```python
from build123d import *

# Parameters (mm, degrees)
SKETCH1_W                      = 96
SKETCH1_H                      = 32
BOSS_EXTRUDE1_DEPTH            = 32
SKETCH2_W                      = 28
SKETCH2_H                      = 30
CUT_EXTRUDE1_DEPTH             = 97
F_8_0_8_DIAMETER_HOLE1_D       = 8
F_8_0_8_DIAMETER_HOLE1_DEPTH   = 2
F_3_7_3_7_DIAMETER_HOLE1_D     = 3.7
F_3_7_3_7_DIAMETER_HOLE1_DEPTH = 2
F_3_7_3_7_DIAMETER_HOLE2_D     = 3.7
F_3_7_3_7_DIAMETER_HOLE2_DEPTH = 32
F_8_0_8_DIAMETER_HOLE2_D       = 8
F_8_0_8_DIAMETER_HOLE2_DEPTH   = 32
F_8_0_8_DIAMETER_HOLE3_D       = 8
F_8_0_8_DIAMETER_HOLE3_DEPTH   = 2
F_8_0_8_DIAMETER_HOLE4_D       = 8
F_8_0_8_DIAMETER_HOLE4_DEPTH   = 32
F_3_7_3_7_DIAMETER_HOLE3_D     = 3.7
F_3_7_3_7_DIAMETER_HOLE3_DEPTH = 32
FILLET1_R                      = 2.5


with BuildPart() as part:
    # Sketch1 → Boss-Extrude1 (new body)
    with BuildSketch(Plane(origin=(16, 0, 0), x_dir=(0, 0, -1), z_dir=(1, 0, 0))):
        with Locations((32, 16)):
            Rectangle(SKETCH1_W, SKETCH1_H)
    extrude(amount=-BOSS_EXTRUDE1_DEPTH)

    # Sketch2 → Cut-Extrude1 (cut, through all)
    with BuildSketch(Plane(origin=(0, 0, -80), x_dir=(-1, 0, 0), z_dir=(0, 0, -1))):
        with Locations((0, 17)):
            Rectangle(SKETCH2_W, SKETCH2_H)
    extrude(amount=-CUT_EXTRUDE1_DEPTH, mode=Mode.SUBTRACT)

    # Ø8.0 (8) Diameter Hole1
    with Locations(Plane.ZY.offset(16)):
        with Locations((-64, 16), (-32, 16), (-16, 16), (-48, 16), (0, 16)):
            Hole(F_8_0_8_DIAMETER_HOLE1_D / 2, depth=F_8_0_8_DIAMETER_HOLE1_DEPTH)

    # Ø3.7 (3.7) Diameter Hole1
    with Locations(Plane.ZY.offset(16)):
        with Locations((0, 24), (0, 8), (-8, 16), (8, 16), (-5.656854249, 21.656854249), (5.656854249, 21.656854249), (5.656854249, 10.343145751), (-5.656854249, 10.343145751), (-64, 24), (-64, 8), (-72, 16), (-56, 16), (-69.656854249, 21.656854249), (-58.343145751, 21.656854249), (-58.343145751, 10.343145751), (-69.656854249, 10.343145751), (-32, 24), (-40, 16), (-32, 8), (-24, 16)):
            Hole(F_3_7_3_7_DIAMETER_HOLE1_D / 2, depth=F_3_7_3_7_DIAMETER_HOLE1_DEPTH)

    # Ø3.7 (3.7) Diameter Hole2
    with Locations(Plane(origin=(0, 0, 0), x_dir=(-1, 0, 0), z_dir=(0, -1, 0))):
        with Locations((8, 0), (5.656854249, 5.656854249), (0, 8), (-5.656854249, 5.656854249), (-8, 0), (-5.656854249, -5.656854249), (0, -8), (5.656854249, -5.656854249), (8, 64), (5.656854249, 69.656854249), (0, 72), (-5.656854249, 69.656854249), (-8, 64), (-5.656854249, 58.343145751), (0, 56), (5.656854249, 58.343145751), (8, 32), (0, 40), (-8, 32), (0, 24)):
            Hole(F_3_7_3_7_DIAMETER_HOLE2_D / 2, depth=F_3_7_3_7_DIAMETER_HOLE2_DEPTH)

    # Ø8.0 (8) Diameter Hole2
    with Locations(Plane(origin=(0, 0, 0), x_dir=(-1, 0, 0), z_dir=(0, -1, 0))):
        with Locations((0, 0), (0, 64), (0, 32), (0, 16), (0, 48)):
            Hole(F_8_0_8_DIAMETER_HOLE2_D / 2, depth=F_8_0_8_DIAMETER_HOLE2_DEPTH)

    # Ø8.0 (8) Diameter Hole3
    with Locations(Plane.ZY.offset(-14)):
        with Locations((-32, 16)):
            Hole(F_8_0_8_DIAMETER_HOLE3_D / 2, depth=F_8_0_8_DIAMETER_HOLE3_DEPTH)

    # Ø8.0 (8) Diameter Hole4
    with Locations(Plane(origin=(16, 0, 0), x_dir=(0, 0, -1), z_dir=(1, 0, 0))):
        with Locations((64, 16), (16, 16), (48, 16), (0, 16)):
            Hole(F_8_0_8_DIAMETER_HOLE4_D / 2, depth=F_8_0_8_DIAMETER_HOLE4_DEPTH)

    # Ø3.7 (3.7) Diameter Hole3
    with Locations(Plane(origin=(16, 0, 0), x_dir=(0, 0, -1), z_dir=(1, 0, 0))):
        with Locations((0, 24), (0, 8), (8, 16), (-8, 16), (5.656854249, 21.656854249), (-5.656854249, 21.656854249), (-5.656854249, 10.343145751), (5.656854249, 10.343145751), (64, 24), (64, 8), (72, 16), (56, 16), (69.656854249, 21.656854249), (58.343145751, 21.656854249), (58.343145751, 10.343145751), (69.656854249, 10.343145751), (32, 24), (40, 16), (32, 8), (24, 16)):
            Hole(F_3_7_3_7_DIAMETER_HOLE3_D / 2, depth=F_3_7_3_7_DIAMETER_HOLE3_DEPTH)

    # Fillet1
    fillet1_edges = [part.edges().sort_by_distance(p)[0] for p in [
        (-16, 0, -32),
        (15, 32, 16),
        (15, 32, -80),
        (16, 0, -32),
        (-15, 32, -80),
        (-15, 32, 16),
    ]]
    fillet(fillet1_edges, radius=FILLET1_R)


solid = part.part
```
CAD build for the part. Positions are in the model's coordinates, mm. Round coordinates to 2 decimals unless told otherwise and drop trailing zeros. Order: outer loops, then holes, each group sorted by start corner. A loop starts at its lowest first (then second) coordinate and runs counter-clockwise, first axis right, second up.
Item 1: Pin check, flat tips, straight feed: pin 1 (5 mm diameter, centred on y = 24, z = 0, fed in from -X); pin 2 (1.5 mm diameter, centred on x = -12.5, z = 4.5, fed in from +Y). Stop position of each tip, or through.
Item 2: Saw through at A-A on z = -40. Write the cut outline in (x, y), then the cut area to 3 significant figures.
Item 3: Saw through at C-C on x = 8.5. Write the cut outline in (y, z), then the cut area to 3 significant figures.
Item 4: Saw through at D-D on z = -64. State how many separate pieces and enclosed holes the cut face has, then the cut area to 3 significant figures.
Item 5: Saw through at B-B on z = -27. Write the cut outline in (x, y).
Item 6: Mould opens along Y. For faces 1 (the face through (-5.898, 1.014, -60.177)), 2 (the face through (15, 32, -31)), 3 (the face through (-14.986, 9.217, 7.125)), 4 (the face through (-14.99, 19.85, 6.06)) say: pulls with the +Y half, pulls with the -Y half, needs draft (parallel to the pull), parting line crosses it, or undercut.
Item 7: Probe line 1 along Z through (x, y) = (-15, 8); line 2 along X through (y, z) = (5, -15.5); line 3 along Y through (x, z) = (14.6, 0) (3 decimals). List the from-to ranges inside material, lowest first.
Reported:
1. pin 1: stops at x = -16
1. pin 2: stops at y = 2
2. outline: (-16, 2.5) arc R2.5 ccw to (-13.5, 0) - (-1.85, 0) - (-1.85, 2) - (-14, 2) - (-14, 14.15) - (-16, 14.15) - close; (-16, 17.85) - (-14, 17.85) - (-14, 32) - (-16, 32) - close; (1.85, 0) - (13.5, 0) arc R2.5 ccw to (16, 2.5) - (16, 14.15) - (14, 14.15) - (14, 2) - (1.85, 2) - close; (14, 17.85) - (16, 17.85) - (16, 32) - (14, 32) - close
2. area: 159 mm2
3. outline: (0, -80) - (2, -80) - (2, -65.78) - (0, -65.78) - close; (0, -62.22) - (2, -62.22) - (2, -33.78) - (0, -33.78) - close; (0, -30.22) - (2, -30.22) - (2, -1.78) - (0, -1.78) - close; (0, 1.78) - (2, 1.78) - (2, 16) - (0, 16) - close
3. area: 171 mm2
4. separate pieces: 10
4. enclosed holes: 0
4. area: 88.9 mm2
5. outline: (-16, 2.5) arc R2.5 ccw to (-13.5, 0) - (13.5, 0) arc R2.5 ccw to (16, 2.5) - (16, 32) - (14, 32) - (14, 2) - (-14, 2) - (-14, 32) - (-16, 32) - close
6. face 1: needs draft
6. face 2: pulls with the +Y half
6. face 3: undercut
6. face 4: undercut
7. line 1: z = -80 to -65.85, -62.15 to -33.85, -30.15 to -1.85, 1.85 to 16
7. line 2: x = -16 to -14, 14 to 16
7. line 3: y = 0.255 to 6.15, 9.85 to 12, 20 to 22.15, 25.85 to 32
